```python
from build123d import *

# Parameters (mm, degrees)
SKETCH_1_W      = 74
SKETCH_1_H      = 7
SKETCH_1_W_2    = 10
SKETCH_1_H_2    = 3
SKETCH_1_W_3    = 3
SKETCH_1_H_3    = 5
EXTRUDE_1_DEPTH = 3


with BuildPart() as part:
    # 草圖1 → 填料-伸長1 (new body)
    with BuildSketch(Plane.XY):
        Polygon((-37, 4), (-37, 3.5), (-9, 3.5), (-9, 6.5), (-37, 6.5), align=None)
        Rectangle(SKETCH_1_W, SKETCH_1_H)
        with Locations((0, 5)):
            Rectangle(SKETCH_1_W_2, SKETCH_1_H_2)
        Polygon((9, 6.5), (9, 3.5), (37, 3.5), (37, 4), (37, 6.5), align=None)
        with Locations((-38.5, 1.5)):
            Rectangle(SKETCH_1_W_3, SKETCH_1_H_3)
        with Locations((38.5, 1.5)):
            Rectangle(SKETCH_1_W_3, SKETCH_1_H_3)
    extrude(amount=EXTRUDE_1_DEPTH)


solid = part.part
```
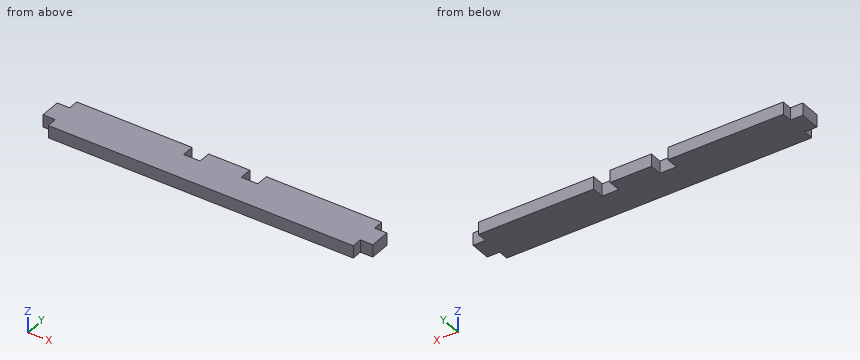
Check sheet for the modelled part. Datum: model origin and axes. Units: mm. Round coordinates to 2 decimals unless told otherwise and drop trailing zeros. Order: outer loops, then holes, each group sorted by start corner. A loop starts at its lowest first (then second) coordinate and runs counter-clockwise, first axis right, second up. Notation, with made-up numbers: (85, 59.25) -> (93, 59.25) arc R17 ccw to (93, 83.25) -> close; hole circle Ø8 at (23.5, 49). An arc over 180 degrees is marked (long way). One line per item, written item: value. Start each with the question number.
Q1. Gauge pin test, flat ends, axial feed: pin 1 Ø1.5 at (x, z) = (7, 1) entering from +Y; pin 2 Ø0.9 at (x, z) = (-39, 2) entering from +Y; pin 3 Ø1.2 at (y, z) = (5.5, 1.5) entering from +X; pin 4 Ø1.5 at (y, z) = (4.5, 1.5) entering from +X. Record the tip position at first contact, or that the pin passes through.
Q2. Cross-section at B-B (z = 1.95). Record the boundary of the cut face in (x, y), and give its area (3 significant figures).
Q3. Cross-section at A-A (y = 5). Record the boundary of the cut face in (x, z).
Q4. Thickness scan on line 1 (X direction, y = 4.5, z = 2.2); line 2 (Y direction, x = 6, z = 0.45); line 3 (X direction, y = -2.75, z = 2.15). Record the ranges inside material, lowest first.
Completed:
1. pin 1: stops at y = 3.5
1. pin 2: stops at y = 4
1. pin 3: stops at x = 37
1. pin 4: stops at x = 40
2. outline: (-40, -1) -> (-37, -1) -> (-37, -3.5) -> (37, -3.5) -> (37, -1) -> (40, -1) -> (40, 4) -> (37, 4) -> (37, 6.5) -> (9, 6.5) -> (9, 3.5) -> (5, 3.5) -> (5, 6.5) -> (-5, 6.5) -> (-5, 3.5) -> (-9, 3.5) -> (-9, 6.5) -> (-37, 6.5) -> (-37, 4) -> (-40, 4) -> close
2. area: 746 mm²
3. outline: (-37, 0) -> (-9, 0) -> (-9, 3) -> (-37, 3) -> close; (-5, 0) -> (5, 0) -> (5, 3) -> (-5, 3) -> close; (9, 0) -> (37, 0) -> (37, 3) -> (9, 3) -> close
4. line 1: x = -37 to -9, -5 to 5, 9 to 37
4. line 2: y = -3.5 to 3.5
4. line 3: x = -37 to 37
